The drawing under review shows one solid part. Ordinate dimensions are in mm from its lowest x, y, z. Give positions to 0.01 mm unless a question says otherwise; leave off trailing zeros. Order: outer loops, then holes, each group sorted by start corner. A loop starts at its lowest first (then second) coordinate and runs counter-clockwise, first axis right, second up. Notation, with made-up numbers: (-26, 87) -> (30, 87) arc R16 cw to (30, 115) -> close; hole circle Ø4 at (-11, -35.5). An arc over 180 degrees is marked (long way). Use a Markdown table: item, result. Add a question column.
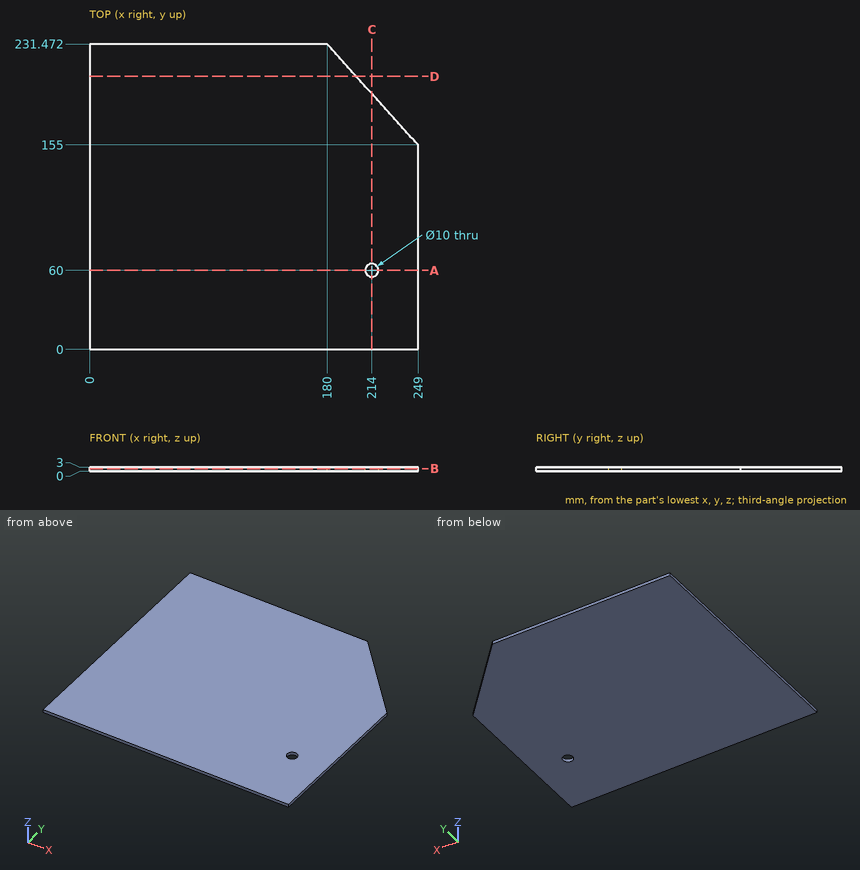
1) Add section D-D (y = 207). Give the boundary of the cut face in (x, z), then the cut area to 3 significant figures.
2) Add section B-B (z = 2.15). Give the boundary of the cut face in (x, y).
3) Add section A-A (y = 60). Give the boundary of the cut face in (x, z).
4) For L1, parallel to Y at x = 214, z = 1.45; L2, parallel to X at y = 199, z = 2.3; L3, parallel to X at y = 166, z = 0.2 (1 decimal), list the stretches that pass through material, from the lowest coordinate up. Write a range as [from, to].
5) Add section C-C (x = 214). Give the boundary of the cut face in (y, z).
Worked answers:
| question | item | result |
|---|---|---|
| 1 | outline | (0, 0) -> (202.08, 0) -> (202.08, 3) -> (0, 3) -> close |
| 1 | area | 606 mm^2 |
| 2 | outline | (0, 0) -> (249, 0) -> (249, 155) -> (180, 231.47) -> (0, 231.47) -> close; hole circle Ø10 at (214, 60) |
| 3 | outline | (0, 0) -> (209, 0) -> (209, 3) -> (0, 3) -> close; (219, 0) -> (249, 0) -> (249, 3) -> (219, 3) -> close |
| 4 | L1 | [0, 55], [65, 193.79] |
| 4 | L2 | [0, 209.3] |
| 4 | L3 | [0, 239.1] |
| 5 | outline | (0, 0) -> (55, 0) -> (55, 3) -> (0, 3) -> close; (65, 0) -> (193.79, 0) -> (193.79, 3) -> (65, 3) -> close |
